Here's how the part is built. I have some questions about the finished solid (model axes, mm). Face numbers are marked on the shaded views. A direction names the side the tool comes from. Round coordinates to 2 decimals unless told otherwise and drop trailing zeros. Loops run counter-clockwise (first coordinate to the right, second up) from the corner with the lowest first, then second, coordinate; pieces in that order, holes last. Notation, with made-up numbers: M -36,4 L 12,4 A22 cw 12,24 Z; hole C -1,68 d1. An arc over 180 degrees is marked long. Use a Markdown table: item, result.
```python
from build123d import *

# Parameters (mm, degrees)
CROQUIS1_R              = 10
SALIENTE_EXTRUIR1_DEPTH = 14
SALIENTE_EXTRUIR2_START = 20
CROQUIS5_R              = 10
SALIENTE_EXTRUIR2_DEPTH = 40


with BuildPart() as part:
    # Croquis1 → Saliente-Extruir1 (new body)
    with BuildSketch(Plane(origin=(0, 0, 0), x_dir=(1, 0, 0), z_dir=(0, 1, 0))):
        with BuildLine():
            Line((0, 0), (80, 0))
            ThreePointArc((80, 0), (110, 30), (80, 60))
            Line((80, 60), (0, 60))
            ThreePointArc((0, 60), (-30, 30), (0, 0))
        make_face()
        with Locations(Location((0, 30, 0), (0, 0, 270))):
            Circle(CROQUIS1_R, mode=Mode.SUBTRACT)
        with Locations(Location((80, 30, 0), (0, 0, 270))):
            Circle(CROQUIS1_R, mode=Mode.SUBTRACT)
    extrude(amount=SALIENTE_EXTRUIR1_DEPTH)

    # Croquis5 → Saliente-Extruir2 (add)
    with BuildSketch(Plane(origin=(0, 0, 0), x_dir=(0, 0, -1), z_dir=(1, 0, 0)).offset(SALIENTE_EXTRUIR2_START)):
        with BuildLine():
            Line((60, 14), (60, 30))
            ThreePointArc((60, 30), (30, 60), (0, 30))
            Line((0, 30), (0, 14))
            Line((0, 14), (60, 14))
        make_face()
        with Locations((30, 30)):
            Circle(CROQUIS5_R, mode=Mode.SUBTRACT)
    extrude(amount=SALIENTE_EXTRUIR2_DEPTH)


solid = part.part
```
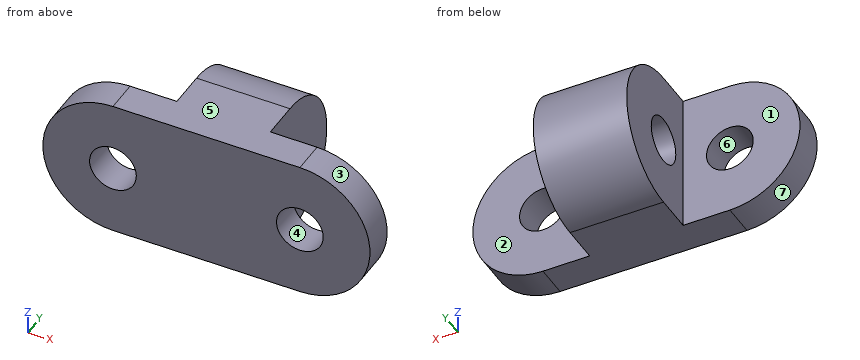
Q1. Will these pins go through, and if not, where does the flat tip stop? P1, Ø10, axis at y = 36, z = -25, coming from the -X side; P2, Ø4, axis at x = -10, z = -30.5, coming from the -Y side; P3, Ø4, axis at x = 43, z = -23.5, coming from the +Y side; P4, Ø6, axis at y = 20.5, z = -21, coming from the +X side.
Return value:
| item | result |
|---|---|
| P1 | stops at x = 20 |
| P2 | stops at y = 0 |
| P3 | stops at y = 59.66 |
| P4 | stops at x = 60 |
Q2. Imagine slicing it at B-B, the plane z = -30. Please give me the cut outline in (x, y).
Return value:
| item | result |
|---|---|
| outline | M -30,0 L -10,0 L -10,14 L -30,14 Z; M 10,0 L 70,0 L 70,14 L 60,14 L 60,20 L 20,20 L 20,14 L 10,14 Z; M 20,40 L 60,40 L 60,60 L 20,60 Z; M 90,0 L 110,0 L 110,14 L 90,14 Z |
Q3. Imagine slicing it at A-A, the plane x = 72. Please give me the cut outline in (y, z), then the cut area to 3 significant figures.
Return value:
| item | result |
|---|---|
| outline | M 0,-60 L 14,-60 L 14,-36 L 0,-36 Z; M 0,-24 L 14,-24 L 14,0 L 0,0 Z |
| area | 672 mm^2 |
Q4. We'd pull the mould along X, two halves only. Please class the marked faces 4, 5, 6 and 7: pulls with the +X half, pulls with the -X half, needs draft (parallel to the pull), parting line crosses it, or undercut.
Return value:
| item | result |
|---|---|
| face 4 | undercut |
| face 5 | needs draft |
| face 6 | undercut |
| face 7 | pulls with the -X half |
Q5. For the marked faces 1, 2 and 3, which set-ups out of +Z, -Z, +X, -X, +Y, -Y let a thin tool reach every point of the face, with its end or its side?
Return value:
| item | result |
|---|---|
| face 1 | +Z, -Z, -X, +Y |
| face 2 | +Z, -Z, +X, +Y |
| face 3 | +X, +Y, -Y |
Q6. Imagine slicing it at C-C, the plane x = 42. Please give me the cut outline in (y, z), then the cut area to 3 significant figures.
Return value:
| item | result |
|---|---|
| outline | M 0,-60 L 30,-60 A30 ccw 30,0 L 0,0 Z; hole C 30,-30 d20 |
| area | 2,900 mm^2 |
Q7. Imagine slicing it at D-D, the plane y = 34. Please give me the cut outline in (x, z).
Return value:
| item | result |
|---|---|
| outline | M 20,-59.73 L 60,-59.73 L 60,-39.17 L 20,-39.17 Z; M 20,-20.83 L 60,-20.83 L 60,-0.27 L 20,-0.27 Z |
Q8. I need wall thicknesses on line 1 (X direction, y = 10.5, z = -30); line 2 (Y direction, x = 44.5, z = -30); line 3 (X direction, y = 3.5, z = -34). Which ranges of each line are inside material? Lowest first, please. Write a range as from..to.
Return value:
| item | result |
|---|---|
| line 1 | x = -30..-10, 10..70, 90..110 |
| line 2 | y = 0..20, 40..60 |
| line 3 | x = -29.73..-9.17, 9.17..70.83, 89.17..109.73 |
